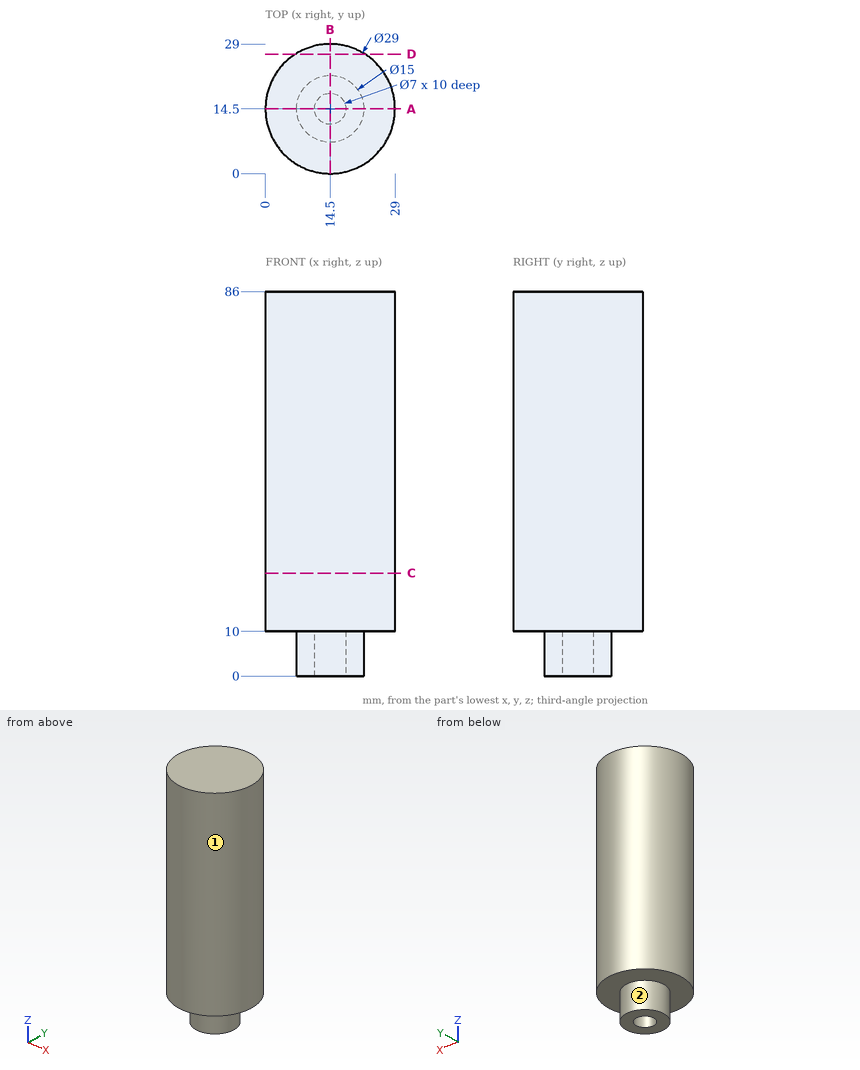
Answer from the drawing. Dimensions are ordinates in mm from the lowest x, y and z of the part. A direction names the side the tool comes from. Coordinates: 2 decimals unless noted, no trailing zeros. Write each loop counter-clockwise with the first axis right and the second up, starting at its lowest first coordinate (ties: lowest second). Pieces come first, ordered by that corner, then holes. Notation, with made-up numbers: (-20, 47.25) - (38, 47.25) arc R16 cw to (38, 66.25) - close; hole circle Ø8 at (76, 20.5). An arc over 180 degrees is marked (long way). Return JSON: item names as keys, results as strings.
1. The part is cut by section C-C on z = 23. Determine the outline of the cut face in (x, y), then the cut area to 3 significant figures.
Final values:
{"outline": "circle Ø29 at (14.5, 14.5)", "area": "661 mm^2"}
2. The part is cut by section A-A on y = 14.5. Determine the outline of the cut face in (x, z).
Final values:
{"outline": "(0, 10) - (7, 10) - (7, 0) - (11, 0) - (11, 10) - (18, 10) - (18, 0) - (22, 0) - (22, 10) - (29, 10) - (29, 86) - (0, 86) - close"}
3. The part is cut by section D-D on y = 26.75. Determine the outline of the cut face in (x, z).
Final values:
{"outline": "(6.74, 10) - (22.26, 10) - (22.26, 86) - (6.74, 86) - close"}
4. Which of the six approach directions +Z, -Z, +X, -X, +Y, -Y give full straight-line access (tool end or side, diameter ignored) to the marked faces 1 and 2?
Final values:
{"face 1": "+Z, -Z", "face 2": "-Z"}
5. Each of these flat-tipped pins is pushed along its axis until it touches: pin 1 Ø4 at (x, z) = (9, 41.5) entering from +Y; pin 2 Ø4 at (x, z) = (11, 45) entering from -Y; pin 3 Ø4 at (y, z) = (5.5, 33) entering from -X. Where does it stop, or does it pass through?
Final values:
{"pin 1": "y = 28.57", "pin 2": "y = 0.08", "pin 3": "x = 1.8"}
6. Consider line 1 along Y through (x, z) = (14.5, 4.5); line 2 along Z through (x, y) = (14, 25.75); line 3 along X through (y, z) = (16.5, 81.5). Determine where each line is inside the solid, lowest interval first.
Final values:
{"line 1": "7 to 11, 18 to 22", "line 2": "10 to 86", "line 3": "0.14 to 28.86"}
